The listing builds one solid part. Answer for the finished solid, in the listing's coordinates (mm). A direction names the side the tool comes from. Give positions to 0.01 mm unless a question says otherwise; leave off trailing zeros. Order: outer loops, then holes, each group sorted by start corner. A loop starts at its lowest first (then second) coordinate and runs counter-clockwise, first axis right, second up. Notation, with made-up numbers: (47, 13) - (84, 13) arc R26 ccw to (84, 40) - close; hole circle Ø1 at (-25, 50.5). An arc over 180 degrees is marked (long way). Use a Markdown table: item, result. Add a question column.
1) Find section B-B, the plane x = 64.75. Determine the outline of the cut face in (y, z).
2) The mould has two halves that part along X. Classify faces 4 (the face through (-1, 0, 1)), 5 (the face through (39.49, 3.25, 26.37)), 6 (the face through (41.4, 6.6, 26.1)): released by +X, released by -X, zero draft, split by the parting line, or undercut.
3) Find section A-A, the plane x = -37.5. Determine the outline of the cut face in (y, z).
4) Flat-ended cylindrical pins translate along their axes: pin 1 (4.5 mm diameter, centred on x = -64.75, z = 25, fed in from +Y); pin 2 (4 mm diameter, centred on x = -64.75, z = -40, fed in from -Y); pin 3 (7 mm diameter, centred on x = -66, z = 40.5, fed in from -Y); pin 4 (1.5 mm diameter, centred on x = 18.5, z = 14.5, fed in from +Y). Find the tip coordinate at first contact, or state that the pin passes through.
5) Straight lines are drawn through the part: line 1 (X direction, y = 7.55, z = -25); line 2 (X direction, y = 2.6, z = 40); line 3 (X direction, y = 4.8, z = 40). For each, find the intervals that lie inside material, in ascending order.
6) Find section D-D, the plane x = 15.25. Determine the outline of the cut face in (y, z), plus the area to 3 significant figures.
7) For faces 1 (the face through (-8, 6.6, -23)), 2 (the face through (-29.75, 5, 0)), 3 (the face through (63.77, 1.72, -43.1)), determine the directions among +Z, -Z, +X, -X, +Y, -Y from which every point of the face is accessible in a straight line to the end or side of a thin tool.
8) Find section C-C, the plane z = 40. Determine the outline of the cut face in (x, y), plus the area to 3 significant figures.
Autodesk Inventor part; units mm, degrees
ref_plane "YZ Plane" through (0, 0, 0) normal (1, 0, 0) x (0, 1, 0)
ref_plane "XZ Plane" through (0, 0, 0) normal (0, 1, 0) x (-1, 0, 0)
ref_plane "XY Plane" through (0, 0, 0) normal (0, 0, 1) x (1, 0, 0)
sketch "Sketch1" plane through (0, 0, 0) normal (0, 1, 0) x (-1, 0, 0)
  line L0 (69.75, 45) -> (-69.75, 45)
  line L1 (-69.75, 45) -> (-69.75, -45)
  line L2 (-69.75, -45) -> (69.75, -45)
  line L3 (69.75, -45) -> (69.75, 45)
  line L4 (69.75, 45) -> (-69.75, -45) construction
  line L5 (-69.75, 45) -> (69.75, -45) construction
  circle A0 centre (44.75, 0) radius 8 construction
  circle A1 centre (-15.25, 0) radius 14.5
  line L6 (152.1746, 0) -> (-152.1746, 0) construction
  line L7 (0, 58.0523) -> (0, -58.0523) construction
  line L8 (29.75, 20) -> (59.75, 20)
  line L9 (59.75, 20) -> (59.75, -20)
  line L10 (59.75, -20) -> (29.75, -20)
  line L11 (29.75, -20) -> (29.75, 20)
  line L12 (29.75, 20) -> (59.75, -20) construction
  line L13 (59.75, 20) -> (29.75, -20) construction
  point P0 (0, 0)
  dimension "d0" = 139.5
  dimension "d1" = 16
  dimension "d2" = 29
  dimension "d3" = 25
  dimension "d4" = 90
  dimension "d5" = 54.5
  dimension "d42" = 30
  dimension "d43" = 40
extrude "Extrusion1" add sketch "Sketch1" along normal blind 10
sketch "Sketch2" plane through (0, 0, 0) normal (0, -1, 0) x (1, 0, 0)
  line L0 (64.75, 40) -> (-64.75, 40) construction
  line L1 (-64.75, 40) -> (-64.75, -40) construction
  line L2 (-64.75, -40) -> (64.75, -40) construction
  line L3 (64.75, -40) -> (64.75, 40) construction
  line L4 (64.75, 40) -> (-64.75, -40) construction
  line L5 (-64.75, 40) -> (64.75, -40) construction
  line L6 (69.75, -45) -> (-69.75, -45) construction
  line L7 (-69.75, -45) -> (-69.75, 45) construction
  point P0 (0, 0)
  dimension "d11" = 5
  dimension "d12" = 5
hole "Hole1" at (64.75, 0, -40) at (-64.75, 0, -40) at (-64.75, 0, 40) at (64.75, 0, 40) direction (0, 1, 0) diameter 3.4 end through all counterbore diameter 6.5 counterbore depth 3.4
sketch "Sketch3" plane through (0, 10, 0) normal (0, 1, 0) x (1, 0, 0)
  circle A0 centre (-64.75, 40) radius 1.7
  circle A1 centre (-64.75, 40) radius 4
  circle A2 centre (64.75, -40) radius 1.7
  circle A3 centre (-64.75, -40) radius 1.7
  circle A4 centre (-64.75, 40) radius 1.7
  circle A5 centre (64.75, 40) radius 1.7
  line L0 (69.75, -45) -> (69.75, 45)
  line L1 (69.75, 45) -> (-69.75, 45)
  line L2 (-69.75, 45) -> (-69.75, -45)
  line L3 (-69.75, -45) -> (69.75, -45)
  circle A6 centre (64.75, 40) radius 4
  circle A7 centre (-64.75, -40) radius 4
  circle A8 centre (64.75, -40) radius 4
  point P0 (0, 0)
  dimension "d22" = 129.5
  dimension "d25" = 80
  dimension "d28" = 8
  dimension "d37" = 90
  dimension "d38" = 139.5
extrude "Extrusion2" cut sketch "Sketch3" against normal blind 1 contours A0 | A1 | A2 | A3 | A5 | A6 | A7 | A8
sketch "Sketch4" plane through (0, 10, 0) normal (0, 1, 0) x (1, 0, 0)
  circle A0 centre (-64.75, 40) radius 4
  line L0 (69.75, -45) -> (69.75, 45)
  line L1 (69.75, 45) -> (-69.75, 45)
  line L2 (-69.75, 45) -> (-69.75, -45)
  line L3 (-69.75, -45) -> (69.75, -45)
  circle A1 centre (15.25, 0) radius 14.5
  circle A2 centre (15.25, 0) radius 17.5
  point P0 (0, 0)
  dimension "d31" = 35
extrude "Extrusion3" cut sketch "Sketch4" against normal blind 5 contours A2
sketch "Sketch5" plane through (0, 0, 0) normal (0, -1, 0) x (1, 0, 0)
  circle A0 centre (15.25, 0) radius 14.5
  line L0 (69.75, 45) -> (69.75, -45)
  line L1 (-69.75, 45) -> (69.75, 45)
  line L2 (-69.75, -45) -> (-69.75, 45)
  line L3 (69.75, -45) -> (-69.75, -45)
  circle A1 centre (64.75, -40) radius 3.25
  circle A2 centre (-64.75, -40) radius 3.25
  circle A3 centre (-64.75, 40) radius 3.25
  circle A4 centre (64.75, 40) radius 3.25
  circle A5 centre (15.25, 0) radius 9
  point P0 (0, 0)
  dimension "d39" = 18
extrude "Extrusion4" add sketch "Sketch5" against normal blind 4 contours A0
fillet "Fillet1" radius 2 8 edges at (-69.75, 5, 45) (69.75, 5, 45) (69.75, 5, -45) (-69.75, 5, -45) (-59.75, 5, 20) (-59.75, 5, -20) (-29.75, 5, -20) (-29.75, 5, 20)
sketch "Sketch7" plane through (0, 10, 0) normal (0, 1, 0) x (1, 0, 0)
  circle A0 centre (15.25, 0) radius 17.5
  line L0 (15.25, 0) -> (53.4324, -38.1824) construction
  line L1 (-97.65, 0) -> (97.65, 0)
  point P0 (0, 0)
  point P1 (39.9987, -24.7487)
  point P2 (39.9987, 24.7487)
  point P3 (-9.4987, 24.7487)
  point P4 (-9.4987, -24.7487)
  dimension "d46" = 35
  dimension "d49" = 360
  dimension "d51" = 45
hole "Hole2" at (39.9987, 10, 24.7487) at (39.9987, 10, -24.7487) at (-9.4987, 10, -24.7487) at (-9.4987, 10, 24.7487) direction (0, -1, 0) diameter 3.4 end through all counterbore diameter 6.5 counterbore depth 3.4
sketch "Sketch9" plane through (0, 10, 0) normal (0, 1, 0) x (1, 0, 0)
  line L0 (-57.75, 20) -> (-31.75, 20) construction
  line L1 (-59.75, -18) -> (-59.75, 18) construction
  line L2 (-31.75, -20) -> (-57.75, -20) construction
  line L3 (-29.75, 18) -> (-29.75, -18) construction
  line L4 (-64.75, 25) -> (-24.75, 25) construction
  line L5 (-24.75, 25) -> (-24.75, -25) construction
  line L6 (-24.75, -25) -> (-64.75, -25) construction
  line L7 (-64.75, -25) -> (-64.75, 25) construction
  point P0 (0, 0)
  dimension "d63" = 5
  dimension "d64" = 5
  dimension "d65" = 5
  dimension "d66" = 5
hole "Hole3" at (-64.75, 10, -25) at (-24.75, 10, -25) at (-24.75, 10, 25) at (-64.75, 10, 25) direction (0, -1, 0) diameter 3.4 end through all counterbore diameter 6.5 counterbore depth 3.4
properties part number "plate for print"
The answers:
| question | item | result |
|---|---|---|
| 1 | outline | (0, -45) - (10, -45) - (10, -44) - (9, -44) - (9, -41.7) - (3.4, -41.7) - (3.4, -43.25) - (0, -43.25) - close; (0, -36.75) - (3.4, -36.75) - (3.4, -38.3) - (9, -38.3) - (9, -36) - (10, -36) - (10, 36) - (9, 36) - (9, 38.3) - (3.4, 38.3) - (3.4, 36.75) - (0, 36.75) - close; (0, 43.25) - (3.4, 43.25) - (3.4, 41.7) - (9, 41.7) - (9, 44) - (10, 44) - (10, 45) - (0, 45) - close |
| 2 | face 4 | zero draft |
| 2 | face 5 | undercut |
| 2 | face 6 | undercut |
| 3 | outline | (0, -45) - (10, -45) - (10, -20) - (0, -20) - close; (0, 20) - (10, 20) - (10, 45) - (0, 45) - close |
| 4 | pin 1 | y = 6.6 |
| 4 | pin 2 | y = 3.4 |
| 4 | pin 3 | y = 0 |
| 4 | pin 4 | y = 5 |
| 5 | line 1 | -69.75 to -68, -61.5 to -28, -21.5 to -12.74, -6.26 to 36.76, 43.24 to 69.75 |
| 5 | line 2 | -69.75 to -68, -61.5 to 61.5, 68 to 69.75 |
| 5 | line 3 | -69.75 to -66.45, -63.05 to 63.05, 66.45 to 69.75 |
| 6 | outline | (0, -45) - (10, -45) - (10, -17.5) - (5, -17.5) - (5, -14.5) - (4, -14.5) - (4, -9) - (0, -9) - close; (0, 9) - (4, 9) - (4, 14.5) - (5, 14.5) - (5, 17.5) - (10, 17.5) - (10, 45) - (0, 45) - close |
| 6 | area | 624 mm2 |
| 7 | face 1 | +Y |
| 7 | face 2 | +Y, -Y |
| 7 | face 3 | -Y |
| 8 | outline | (-69.75, 0) - (-68, 0) - (-68, 3.4) - (-66.45, 3.4) - (-66.45, 9) - (-68.75, 9) - (-68.75, 10) - (-69.75, 10) - close; (-63.05, 3.4) - (-61.5, 3.4) - (-61.5, 0) - (61.5, 0) - (61.5, 3.4) - (63.05, 3.4) - (63.05, 9) - (60.75, 9) - (60.75, 10) - (-60.75, 10) - (-60.75, 9) - (-63.05, 9) - close; (66.45, 3.4) - (68, 3.4) - (68, 0) - (69.75, 0) - (69.75, 10) - (68.75, 10) - (68.75, 9) - (66.45, 9) - close |
| 8 | area | 1,300 mm2 |
